```python
from build123d import *

# Parameters (mm, degrees)
F1_DEPTH = 9.525
F2_T     = -1.27
F4_DEPTH = 12.7
F5_R     = 1.905
F6_DEPTH = 1.778
F5_R_2   = 6.731
F7_DEPTH = 13.971


with BuildPart() as f1:
    # F0 (on Top) → F1 (new body)
    with BuildSketch(Plane.XY):
        with BuildLine():
            ThreePointArc((-28.0514923582, 7.974917758), (-26.9448485688, 2.4767408919), (-21.9129141613, 0))
            Line((-21.9129141613, 0), (21.9129141613, 0))
            ThreePointArc((21.9129141613, 0), (26.9448485688, 2.4767408919), (28.0514923582, 7.974917758))
            ThreePointArc((28.0514923582, 7.974917758), (23.7696669498, 31.453129083), (15.875, 53.975))
            ThreePointArc((15.875, 53.975), (0, 58.0415066874), (-15.875, 53.975))
            ThreePointArc((-15.875, 53.975), (-23.7696669498, 31.453129083), (-28.0514923582, 7.974917758))
        make_face()
    extrude(amount=F1_DEPTH)

    # F2
    f2_openings = [f1.faces().sort_by_distance(p)[0] for p in [
        (0, 25.796964, 9.525),
    ]]
    offset(amount=F2_T, openings=f2_openings, kind=Kind.INTERSECTION)

    # F3 (on face) → F4 (join)
    with BuildSketch(Plane.XY.offset(1.27)):
        with BuildLine():
            Line((16.4958264334, 21.2362016904), (5.9172176222, 48.402988853))
            ThreePointArc((5.9172176222, 48.402988853), (0, 52.4488543928), (-5.9172176222, 48.402988853))
            Line((-5.9172176222, 48.402988853), (-16.4958263497, 21.2362019052))
            ThreePointArc((-16.4958263497, 21.2362019052), (-15.4827586809, 12.4038814256), (-7.62, 8.255))
            Line((-7.62, 8.255), (7.62, 8.255))
            ThreePointArc((7.62, 8.255), (15.4827586158, 12.4038813304), (16.4958264334, 21.2362016904))
        make_face()
    extrude(amount=F4_DEPTH)

    # F5 (on face) → F6 (join)
    with BuildSketch(Plane.XY.offset(13.97)):
        with Locations((0, 46.0988543928)):
            Circle(F5_R)
        with Locations((-12.065, 15.24)):
            Circle(F5_R)
        with Locations((12.065, 15.24)):
            Circle(F5_R)
    extrude(amount=F6_DEPTH)

    # F5 (on face) → F7 (cut, through all)
    with BuildSketch(Plane.XY.offset(13.97)):
        with Locations((0, 28.575)):
            Circle(F5_R_2)
    extrude(amount=-F7_DEPTH, mode=Mode.SUBTRACT)


solid = f1.part
```
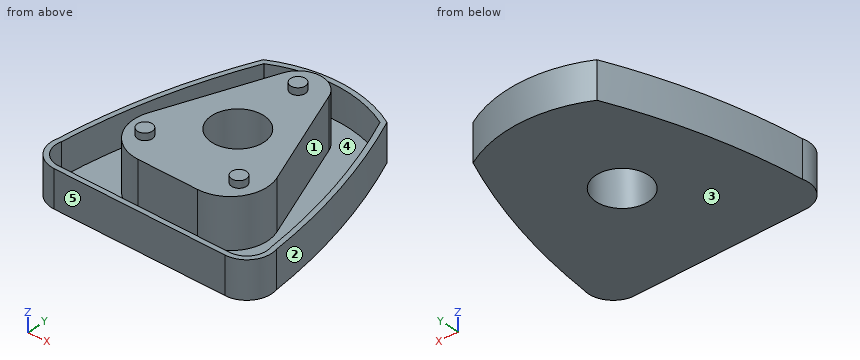
The listing builds one solid part. Answer for the finished solid, in the listing's coordinates (mm). Face numbers are marked on the shaded views. A direction names the side the tool comes from. Round coordinates to 2 decimals unless told otherwise and drop trailing zeros. Order: outer loops, then holes, each group sorted by start corner. A loop starts at its lowest first (then second) coordinate and runs counter-clockwise, first axis right, second up. Notation, with made-up numbers: (36.5, 61) -> (90.5, 61) arc R18 ccw to (90.5, 91) -> close; hole circle Ø2 at (37.25, 65.25). An arc over 180 degrees is marked (long way). Answer as CSV lines item,"result". Start each with the question number.
(1) The part is cut by section B-B (y = 27.5). Determine the outline of the cut face in (x, z) (3 decimals), then the cut area to 3 significant figures.
(2) The part is cut by section D-D (y = 15.24). Determine the outline of the cut face in (x, z) (3 decimals), then the cut area to 3 significant figures.
(3) The part is cut by section A-A (x = 0). Determine the outline of the cut face in (y, z) (1 decimal), then the cut area to 3 significant figures.
(4) For a pull along Y with two mould halves and no side action, classify the marked faces 1, 2 and 3 as +Y half, -Y half, draft (parallel to the pull), parting line (faces both ways), or undercut.
(5) A tool of negligible diameter and unlimited length cuts with its end or side. For the marked faces 4 and 5, from which of +Z, -Z, +X, -X, +Y, -Y can it reach the whole face along a straight path? Write none if from no direction.
(6) The part is cut by section C-C (z = 7). Count the separate pieces of the cut face and the enclosed holes in it, then the cut area to 3 significant figures.
(7) Find the intervals of material crossed by probe 1 along X at (y, z) = (40, 3); probe 2 along X at (y, z) = (24, 9.25) (3 decimals); probe 3 along X at (y, z) = (49, 4), in increasing order. Write a range as from..to.
(8) Flat-ended cylindrical pins translate along their axes: pin 1 Ø6 at (y, z) = (32.5, 10) entering from -X; pin 2 Ø1.5 at (y, z) = (45.5, 2.5) entering from +X; pin 3 Ø3 at (y, z) = (42.5, 2) entering from +X; pin 4 Ø12 at (x, y) = (0, 28.575) entering from +Z. Find the tip coordinate at first contact, or state that the pin passes through.
Evaluation:
1,outline,"(-24.76, 0) -> (-6.645, 0) -> (-6.645, 13.97) -> (-14.057, 13.97) -> (-14.057, 1.27) -> (-23.454, 1.27) -> (-23.454, 9.525) -> (-24.76, 9.525) -> close; (6.645, 0) -> (24.76, 0) -> (24.76, 9.525) -> (23.454, 9.525) -> (23.454, 1.27) -> (14.057, 1.27) -> (14.057, 13.97) -> (6.645, 13.97) -> close"
1,area,"256 mm²"
2,outline,"(-27.131, 0) -> (27.131, 0) -> (27.131, 9.525) -> (25.846, 9.525) -> (25.846, 1.27) -> (16.8, 1.27) -> (16.8, 13.97) -> (13.97, 13.97) -> (13.97, 15.748) -> (10.16, 15.748) -> (10.16, 13.97) -> (-10.16, 13.97) -> (-10.16, 15.748) -> (-13.97, 15.748) -> (-13.97, 13.97) -> (-16.8, 13.97) -> (-16.8, 1.27) -> (-25.846, 1.27) -> (-25.846, 9.525) -> (-27.131, 9.525) -> close"
2,area,"530 mm²"
3,outline,"(0, 0) -> (21.8, 0) -> (21.8, 14) -> (8.3, 14) -> (8.3, 1.3) -> (1.3, 1.3) -> (1.3, 9.5) -> (0, 9.5) -> close; (35.3, 0) -> (58, 0) -> (58, 9.5) -> (56.8, 9.5) -> (56.8, 1.3) -> (52.4, 1.3) -> (52.4, 14) -> (48, 14) -> (48, 15.7) -> (44.2, 15.7) -> (44.2, 14) -> (35.3, 14) -> close"
3,area,"475 mm²"
4,face 1,"undercut"
4,face 2,"+Y half"
4,face 3,"draft"
5,face 4,"+Z"
5,face 5,"+Z, -Z, +X, -X, -Y"
6,separate pieces,"2"
6,enclosed holes,"2"
6,area,"1,150 mm²"
7,probe 1,"-21.24..-19.9, -9.19..9.19, 19.9..21.24"
7,probe 2,"-25.543..-24.245, -15.42..-4.937, 4.937..15.42, 24.245..25.543"
7,probe 3,"-17.97..-16.6, -5.65..5.65, 16.6..17.97"
8,pin 1,"x = -24.26"
8,pin 2,"x = 19.59"
8,pin 3,"x = 20.91"
8,pin 4,"through"
